```python
from build123d import *

# Parameters (mm, degrees)
F4_D = 5


with BuildPart() as f2:
    # F0 (on Front) → F2 (revolve)
    with BuildSketch(Plane.XZ):
        with BuildLine():
            Line((6.5, 50.012508), (6.5, 0))
            Line((6.5, 0), (16, 0))
            Line((16, 0), (16, 24.341691))
            Line((16, 24.341691), (26, 24.341691))
            Line((26, 24.341691), (26, 34.341691))
            Line((26, 34.341691), (16, 34.341691))
            Line((16, 34.341691), (16, 60))
            ThreePointArc((16, 60), (9.254312, 56.904532), (6.5, 50.012508))
        make_face()
    revolve(axis=Axis((0, 0, 35.208348), (0, 0, 1)))

    # F4 (through all)
    with Locations(Plane.XY.offset(34.341691)):
        with Locations((-22.5, 0), (22.5, 0)):
            Hole(F4_D / 2)


solid = f2.part
```
Part model, mm, in its own coordinate system. A direction names the side the tool comes from. Round coordinates to 2 decimals unless told otherwise and drop trailing zeros. Loops run counter-clockwise (first coordinate to the right, second up) from the corner with the lowest first, then second, coordinate; pieces in that order, holes last. Notation, with made-up numbers: (48, 21) -> (99, 21) arc R14 ccw to (99, 27) -> close; hole circle Ø3 at (48, -3). An arc over 180 degrees is marked (long way). Use a Markdown table: item, result.
1) Cut at C-C, the plane z = 38. List the corners of the cut face in (x, y), and give its area (3 significant figures).
The answers:
| item | result |
|---|---|
| outline | circle Ø32 at (0, 0); hole circle Ø13 at (0, 0) |
| area | 672 mm2 |
2) Cut at A-A, the plane y = 0. List the corners of the cut face in (x, z).
The answers:
| item | result |
|---|---|
| outline | (-26, 24.34) -> (-25, 24.34) -> (-25, 34.34) -> (-26, 34.34) -> close; (-20, 24.34) -> (-16, 24.34) -> (-16, 0) -> (-6.5, 0) -> (-6.5, 50.01) arc R10 ccw to (-16, 60) -> (-16, 34.34) -> (-20, 34.34) -> close; (6.5, 0) -> (16, 0) -> (16, 24.34) -> (20, 24.34) -> (20, 34.34) -> (16, 34.34) -> (16, 60) arc R10 ccw to (6.5, 50.01) -> close; (25, 24.34) -> (26, 24.34) -> (26, 34.34) -> (25, 34.34) -> close |
3) Drop flat-ended pins along their axis: pin 1 Ø17 at (x, y) = (0, 0) entering from +Z; pin 2 Ø12 at (x, y) = (2, -9.5) entering from +Z; pin 3 Ø8 at (x, z) = (-0.5, 11.5) entering from -Y. Give the stop position or say it passes through.
The answers:
| item | result |
|---|---|
| pin 1 | stops at z = 56.01 |
| pin 2 | stops at z = 59.98 |
| pin 3 | stops at y = -16 |
4) Cut at B-B, the plane x = 0. List the corners of the cut face in (y, z), and give its area (3 significant figures).
The answers:
| item | result |
|---|---|
| outline | (-26, 24.34) -> (-16, 24.34) -> (-16, 0) -> (-6.5, 0) -> (-6.5, 50.01) arc R10 ccw to (-16, 60) -> (-16, 34.34) -> (-26, 34.34) -> close; (6.5, 0) -> (16, 0) -> (16, 24.34) -> (26, 24.34) -> (26, 34.34) -> (16, 34.34) -> (16, 60) arc R10 ccw to (6.5, 50.01) -> close |
| area | 1,300 mm2 |
5) Pull direction Y, two halves, no side cores. Call faces 3 (the flat face through (11, 12, 34.342)), 4 (the cylindrical face through (-3.47, -15.62, 47.35)), 5 (the cylindrical face through (-20, 0, 29)): pulls with the +Y half, pulls with the -Y half, needs draft (parallel to the pull), parting line crosses it, or undercut.
The answers:
| item | result |
|---|---|
| face 3 | needs draft |
| face 4 | parting line crosses it |
| face 5 | undercut |
6) Cut at D-D, the plane x = 22.5. List the corners of the cut face in (y, z).
The answers:
| item | result |
|---|---|
| outline | (-13.03, 24.34) -> (-2.5, 24.34) -> (-2.5, 34.34) -> (-13.03, 34.34) -> close; (2.5, 24.34) -> (13.03, 24.34) -> (13.03, 34.34) -> (2.5, 34.34) -> close |
7) Tool access for faces 1 (the cylindrical face through (25, 0, 29)), 2 (the cylindrical face through (-3.47, -15.62, 12.34)): list every direction of +Z, -Z, +X, -X, +Y, -Y with a clear straight run to the whole face (end or side of a thin tool).
The answers:
| item | result |
|---|---|
| face 1 | +Z, -Z |
| face 2 | -Z |
8) Probe line 1 (Y direction, x = 0, z = 39); line 2 (Z direction, x = 14.5, y = 17); line 3 (Y direction, x = 0, z = 32). List the from-to ranges inside material, lowest first. Write a range as [from, to].
The answers:
| item | result |
|---|---|
| line 1 | y = [-16, -6.5], [6.5, 16] |
| line 2 | z = [24.34, 34.34] |
| line 3 | y = [-26, -6.5], [6.5, 26] |
